```python
from build123d import *

# Parameters (mm, degrees)
BOSS_EXTRUDE1_DEPTH                                 = 12.7
CSK_FOR_1_4_FLAT_HEAD_MACHINE_SCREW_100_D           = 6.7564
CSK_FOR_1_4_FLAT_HEAD_MACHINE_SCREW_100_CSINK_D     = 12.8778
CSK_FOR_1_4_FLAT_HEAD_MACHINE_SCREW_100_CSINK_ANGLE = 100
FILLET1_R                                           = 6.35


with BuildPart() as part:
    # Sketch1 → Boss-Extrude1 (new body)
    with BuildSketch(Plane.XY):
        with BuildLine():
            Line((0, 0), (0, 43.753600343))
            Line((0, 43.753600343), (-12.7, 43.753600343))
            ThreePointArc((-12.7, 43.753600343), (-20.061287028, 46.138664723), (-24.625181908, 52.3875))
            Line((-24.625181908, 52.3875), (-47.625, 52.3875))
            Line((-47.625, 52.3875), (-47.625, 42.8625))
            Line((-47.625, 42.8625), (-32.935820687, 42.8625))
            ThreePointArc((-32.935820687, 42.8625), (-29.120714859, 41.282231424), (-27.540446284, 37.467125597))
            Line((-27.540446284, 37.467125597), (-27.540446284, 14.840446284))
            ThreePointArc((-27.540446284, 14.840446284), (-23.193780203, 4.346666081), (-12.7, 0))
            Line((-12.7, 0), (0, 0))
        make_face()
    extrude(amount=BOSS_EXTRUDE1_DEPTH)

    # CSK for 1/4 Flat Head Machine Screw (100)1 (through all)
    with Locations(Plane(origin=(0, 52.3875, 0), x_dir=(1, 0, 0), z_dir=(0, 1, 0))):
        with Locations((-41.2242, -6.35)):
            CounterSinkHole(CSK_FOR_1_4_FLAT_HEAD_MACHINE_SCREW_100_D / 2, CSK_FOR_1_4_FLAT_HEAD_MACHINE_SCREW_100_CSINK_D / 2, counter_sink_angle=CSK_FOR_1_4_FLAT_HEAD_MACHINE_SCREW_100_CSINK_ANGLE)

    # Fillet1
    fillet1_edges = [part.edges().sort_by_distance(p)[0] for p in [
        (-47.625, 47.625, 0),
        (-47.625, 47.625, 12.7),
    ]]
    fillet(fillet1_edges, radius=FILLET1_R - 0.0001)  # a hair under: the kernel refuses the full size


solid = part.part
```
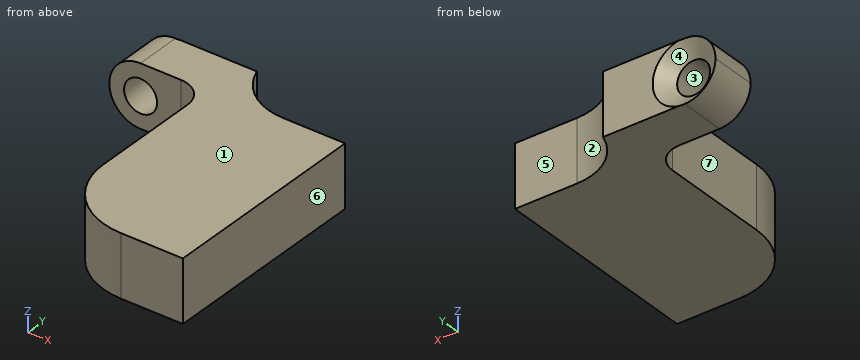
Geometry check sheet. Reference: the model listing, model coordinates, mm. Face numbers are marked on the shaded views. A direction names the side the tool comes from. Round coordinates to 2 decimals unless told otherwise and drop trailing zeros. Order: outer loops, then holes, each group sorted by start corner. A loop starts at its lowest first (then second) coordinate and runs counter-clockwise, first axis right, second up. Notation, with made-up numbers: (87.5, -32.5) - (93.5, -32.5) arc R31 ccw to (93.5, -4.5) - close; hole circle Ø6 at (55, -23.5). An arc over 180 degrees is marked (long way). Use a Markdown table: item, result. Add a question column.
1) Gauge pin test, flat ends, axial feed: P1, Ø2, axis at y = 44, z = 7.5, coming from the -X side; P2, Ø4, axis at x = -6, z = 9, coming from the +Y side; P3, Ø4, axis at y = 22.5, z = 4, coming from the -X side. Record the tip position at first contact, or that the pin passes through.
2) Section check A-A (y = 36). Record the cut outline in (x, z), then the cut area to 3 significant figures.
3) Thickness scan on line 1 along Y through (x, z) = (-6.5, 2); line 2 along X through (y, z) = (17.5, 9.75); line 3 along X through (y, z) = (46.5, 7). Record the ranges inside material, lowest first.
4) Mould release check, pull along Z, two halves, no side actions. Record for the marked faces 1, 2, 3 and 4: released by +Z, released by -Z, zero draft, split by the parting line, or undercut.
5) Section check B-B (x = -30). Record the cut outline in (y, z).
6) Set-up check for the marked faces 5, 6 and 7: record each of +Z, -Z, +X, -X, +Y, -Y from which the full face is reachable in a straight line by a thin tool's end or side.
Established:
| question | item | result |
|---|---|---|
| 1 | P1 | x = -47.62 |
| 1 | P2 | y = 43.75 |
| 1 | P3 | x = -27.54 |
| 2 | outline | (-27.54, 0) - (0, 0) - (0, 12.7) - (-27.54, 12.7) - close |
| 2 | area | 350 mm2 |
| 3 | line 1 | 0 to 43.75 |
| 3 | line 2 | -27.54 to 0 |
| 3 | line 3 | -47.59 to -44.54, -37.91 to -20.54 |
| 4 | face 1 | released by +Z |
| 4 | face 2 | zero draft |
| 4 | face 3 | undercut |
| 4 | face 4 | undercut |
| 5 | outline | (41.99, 0) - (52.39, 0) - (52.39, 12.7) - (41.99, 12.7) - close |
| 6 | face 5 | +Z, -Z, +X, +Y |
| 6 | face 6 | +Z, -Z, +X, +Y, -Y |
| 6 | face 7 | +Z, -Z, -X, -Y |
